Check sheet for the drawn part. Datum: minimum x, y, z corner. Units: mm. A direction names the side the tool comes from. Give positions to 0.01 mm unless a question says otherwise; leave off trailing zeros. Loops run counter-clockwise (first coordinate to the right, second up) from the corner with the lowest first, then second, coordinate; pieces in that order, holes last. Notation, with made-up numbers: (48.25, 88) - (95.25, 88) arc R19 ccw to (95.25, 95) - close; hole circle Ø10 at (-27.5, 50). An arc over 180 degrees is marked (long way). One line per item, written item: value. Start each with the question number.
1. Sectioned sample at C-C (y = 12). Record the cut outline in (x, z), plus the area to 3 significant figures.
2. Scan lines: L1, parallel to Y at x = 47, z = 11.5; L2, parallel to X at y = 13.5, z = 35.5; L3, parallel to Z at x = 27, y = 19.5. Record each from-to range of solid material in increasing order. Write a range as [from, to].
3. Sectioned sample at B-B (x = 31.5). Record the cut outline in (y, z), plus the area to 3 significant figures.
4. Access from +Z, -Z, +X, -X, +Y, -Y to the whole of each face (thin tool, end or side, straight path). Record for the marked faces 1 and 2.
5. Gauge pin test, flat ends, axial feed: pin 1 (3 mm diameter, centred on x = 46.5, z = 23.5, fed in from -Y); pin 2 (17.5 mm diameter, centred on x = 28.38, z = 28.38, fed in from +Y); pin 3 (1.5 mm diameter, centred on x = 26.5, y = 4, fed in from +Z); pin 4 (1.5 mm diameter, centred on y = 4.5, z = 31.5, fed in from +X). Record the tip position at first contact, or that the pin passes through.
6. Sectioned sample at D-D (x = 52). Record the cut outline in (y, z).
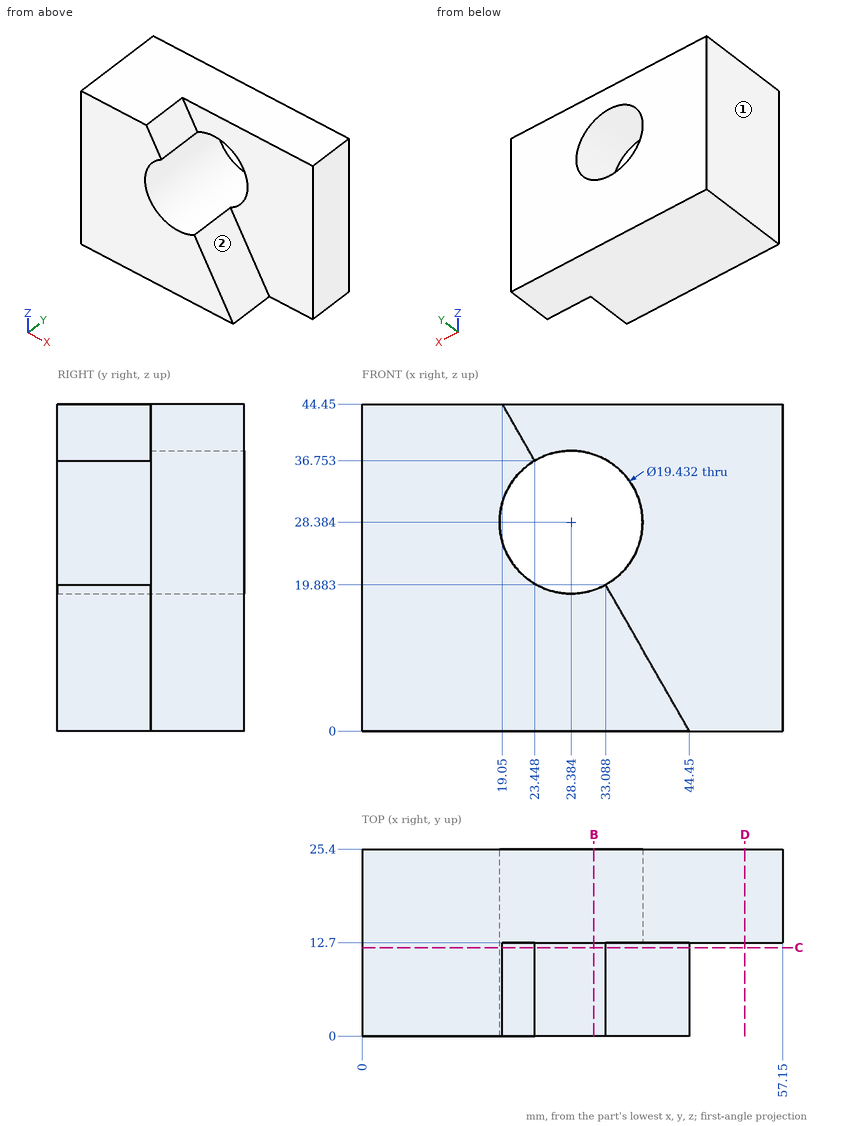
Results are:
1. outline: (0, 0) - (44.45, 0) - (33.09, 19.88) arc R9.72 cw to (23.45, 36.75) - (19.05, 44.45) - (0, 44.45) - close
1. area: 1,270 mm^2
2. L1: y = [12.7, 25.4]
2. L2: x = [0, 21.77], [35, 57.15]
2. L3: z = [0, 18.77], [38, 44.45]
3. outline: (0, 0) - (25.4, 0) - (25.4, 19.18) - (0, 19.18) - close; (12.7, 37.59) - (25.4, 37.59) - (25.4, 44.45) - (12.7, 44.45) - close
3. area: 574 mm^2
4. face 1: +Z, -Z, -X, +Y, -Y
4. face 2: +Z, +X, -Y
5. pin 1: stops at y = 12.7
5. pin 2: passes through
5. pin 3: stops at z = 19.03
5. pin 4: stops at x = 19.47
6. outline: (12.7, 0) - (25.4, 0) - (25.4, 44.45) - (12.7, 44.45) - close
